For this review, use the dimensioned drawing (mm, ordinates from the lowest corner) and the shaded views. Round coordinates to 2 decimals unless told otherwise and drop trailing zeros. Loops run counter-clockwise (first coordinate to the right, second up) from the corner with the lowest first, then second, coordinate; pieces in that order, holes last. Notation, with made-up numbers: M 87.25,44.25 L 112.25,44.25 A29 cw 112.25,65.25 Z; hole C 25,-34 d11. An arc over 180 degrees is marked long. Answer as a JSON object with one key per item and string values. Group by question number.
Item 1: The part is to be moulded in two halves that separate along X. For the marked faces 1, 2 and 3, say which applies: +X half, -X half, draft (parallel to the pull), parting line (faces both ways), or undercut.
Item 2: Consider section D-D (z = 78.5). Give the boundary of the cut face in (x, y).
Item 3: Consider section A-A (x = 19.05). Give the boundary of the cut face in (y, z), and give its area (3 significant figures).
Item 4: To check wall thickness, follow line 1 (Y direction, x = 19.05, z = 34); line 2 (Y direction, x = 19.05, z = 70). State the ranges of each line that lie inside material, in increasing order.
Item 5: Insertion check: P1, Ø6, axis at x = 31, z = 22, coming from the -Y side; P2, Ø12, axis at y = 9, z = 13, coming from the +X side; P3, Ø4, axis at y = 21.5, z = 65.5, coming from the -X side. Each pin has a flat end and moves straight along its axis. Give the tip position at first contact, or say it passes through.
Item 6: Consider section C-C (z = 50.5). Give the boundary of the cut face in (x, y), and give its area (3 significant figures).
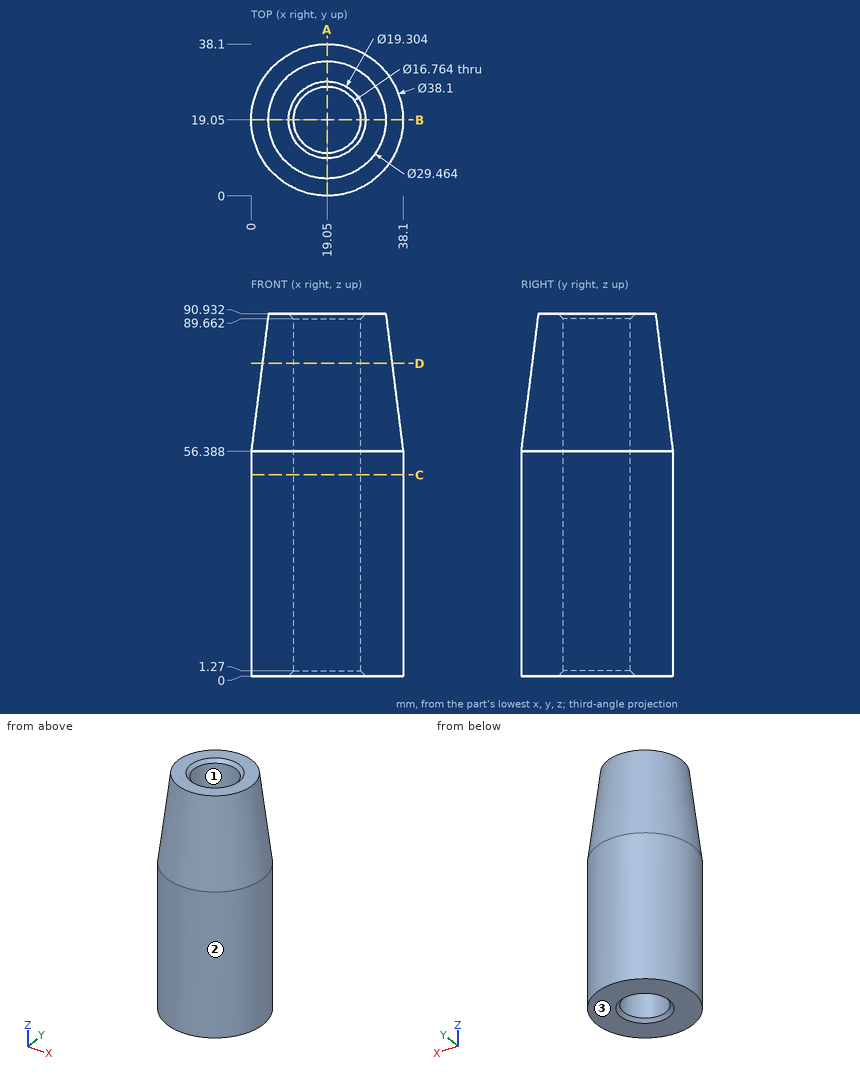
Geometry results:
{
 "1": {"face 1": "undercut", "face 2": "parting line", "face 3": "draft"},
 "2": {"outline": "C 19.05,19.05 d32.57; hole C 19.05,19.05 d16.76"},
 "3": {"outline": "M 0,0 L 9.4,0 L 10.67,1.27 L 10.67,89.66 L 9.4,90.93 L 4.32,90.93 L 0,56.39 Z; M 27.43,1.27 L 28.7,0 L 38.1,0 L 38.1,56.39 L 33.78,90.93 L 28.7,90.93 L 27.43,89.66 Z", "area": "1,790 mm^2"},
 "4": {"line 1": "y = 0 to 10.67, 27.43 to 38.1", "line 2": "y = 1.7 to 10.67, 27.43 to 36.4"},
 "5": {"P1": "stops at y = 2.23", "P2": "stops at x = 37.66", "P3": "stops at x = 0.98"},
 "6": {"outline": "C 19.05,19.05 d38.1; hole C 19.05,19.05 d16.76", "area": "919 mm^2"}
}
